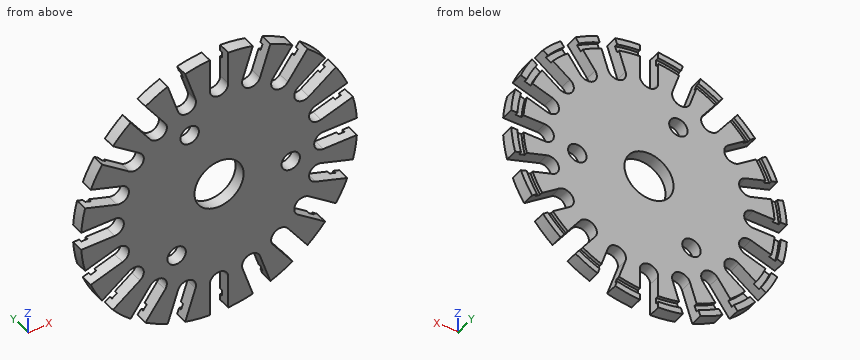
```python
from build123d import *

# Parameters (mm, degrees)
SKETCH1_R           = 22.5
BOSS_EXTRUDE1_DEPTH = 2
CUT_EXTRUDE1_DEPTH  = 2
CIRPATTERN1_COUNT   = 20
SKETCH3_R           = 21.5
SKETCH3_R_2         = 20.5
CUT_EXTRUDE2_DEPTH  = 0.5
SKETCH4_R           = 4
CUT_EXTRUDE3_DEPTH  = 3
SKETCH5_R           = 1.5
CUT_EXTRUDE4_DEPTH  = 10


with BuildPart() as part:
    # Sketch1 → Boss-Extrude1 (new body)
    with BuildSketch(Plane(origin=(0, 0, 0), x_dir=(1, 0, 0), z_dir=(0, 1, 0))):
        Circle(SKETCH1_R)
    extrude(amount=BOSS_EXTRUDE1_DEPTH)

    # Sketch2 → Cut-Extrude1 (cut)
    with BuildSketch(Plane(origin=(0, 2, 0), x_dir=(1, 0, 0), z_dir=(0, 1, 0))):
        with BuildLine():
            Line((1.5, 22.795822005), (1.5, 17))
            ThreePointArc((1.5, 17), (0, 15.5), (-1.5, 17))
            Line((-1.5, 17), (-1.5, 22.795822005))
            ThreePointArc((-1.5, 22.795822005), (0, 24.295822005), (1.5, 22.795822005))
        make_face()
    cut_extrude1 = extrude(amount=-CUT_EXTRUDE1_DEPTH, mode=Mode.SUBTRACT)

    # CirPattern1: Cut-Extrude1 ×20 about axis
    cirpattern1_axis = Axis((0, 0, 0), (0, 1, 0))
    for i in range(1, CIRPATTERN1_COUNT):
        add(cut_extrude1.rotate(cirpattern1_axis, i * 360 / CIRPATTERN1_COUNT), mode=Mode.SUBTRACT)

    # Sketch3 → Cut-Extrude2 (cut)
    with BuildSketch(Plane(origin=(0, 2, 0), x_dir=(1, 0, 0), z_dir=(0, 1, 0))):
        Circle(SKETCH3_R)
        Circle(SKETCH3_R_2, mode=Mode.SUBTRACT)
    extrude(amount=-CUT_EXTRUDE2_DEPTH, mode=Mode.SUBTRACT)

    # Sketch4 → Cut-Extrude3 (cut, through all)
    with BuildSketch(Plane(origin=(0, 2, 0), x_dir=(1, 0, 0), z_dir=(0, 1, 0))):
        Circle(SKETCH4_R)
    extrude(amount=-CUT_EXTRUDE3_DEPTH, mode=Mode.SUBTRACT)

    # Sketch5 → Cut-Extrude4 (cut)
    with BuildSketch(Plane.XZ):
        with Locations((-4.779155556, 10.734159127)):
            Circle(SKETCH5_R)
        with Locations((11.685632271, -1.228209443)):
            Circle(SKETCH5_R)
        with Locations((-6.906476714, -9.505949684)):
            Circle(SKETCH5_R)
    extrude(amount=-CUT_EXTRUDE4_DEPTH, mode=Mode.SUBTRACT)


solid = part.part
```
Build history of the part. All positions in model axes, mm. Round coordinates to 2 decimals unless told otherwise and drop trailing zeros. Order: outer loops, then holes, each group sorted by start corner. A loop starts at its lowest first (then second) coordinate and runs counter-clockwise, first axis right, second up. Notation, with made-up numbers: (79, -15) - (117, -15) arc R26 cw to (117, 18) - close; hole circle Ø4 at (3, 57). An arc over 180 degrees is marked (long way). Use a Markdown table: item, result.
1) Saw through at A-A on x = 0. Write the cut outline in (y, z), and give its area (3 significant figures).
Recorded:
| item | result |
|---|---|
| outline | (0, -15.5) - (2, -15.5) - (2, -4) - (0, -4) - close; (0, 4) - (2, 4) - (2, 15.5) - (0, 15.5) - close |
| area | 46.0 mm² |
2) Wall check: L1, parallel to Z at x = -9.5, y = 0.4; L2, parallel to X at y = 1.8, z = -5; L3, parallel to Z at x = -9, y = 1.05. Give the ranges that are in metal, low to high.
Recorded:
| item | result |
|---|---|
| L1 | z = -20.4 to -15.63, -12.34 to 12.34, 15.63 to 20.4 |
| L2 | x = -21.94 to -20.91, -14.69 to 14.69, 20.91 to 21.94 |
| L3 | z = -20.62 to -14.94, -12.63 to 12.63, 14.94 to 20.62 |
3) Saw through at B-B on y = 0.85. Give the number of separate pieces and of enclosed holes in the cut face, and give its area (3 significant figures).
Recorded:
| item | result |
|---|---|
| separate pieces | 1 |
| enclosed holes | 4 |
| area | 1,120 mm² |
